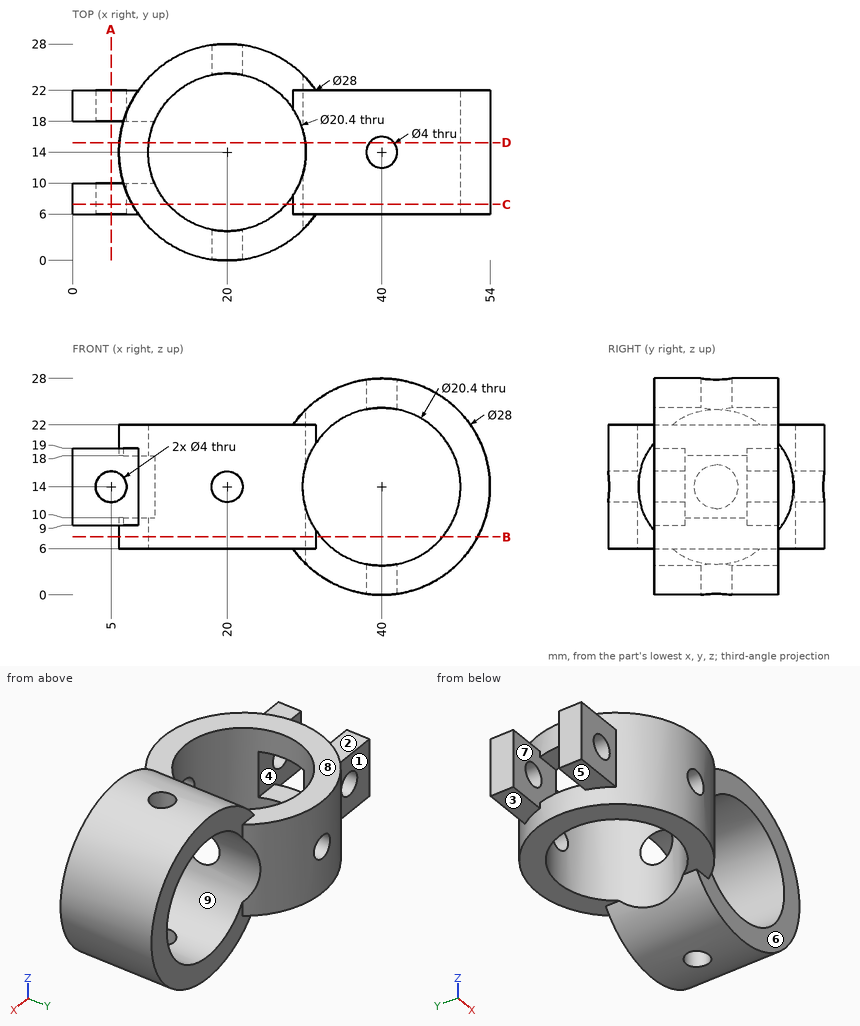
Geometry: see drawing. Coordinates: mm, zero at the bounding-box minimum. A direction names the side the tool comes from. Coordinates: 2 decimals unless noted, no trailing zeros. Loops run counter-clockwise (first coordinate to the right, second up) from the corner with the lowest first, then second, coordinate; pieces in that order, holes last. Notation, with made-up numbers: M 8,20.5 L 47,20.5 A16 cw 47,41.5 Z; hole C 2,22.25 d11. An arc over 180 degrees is marked long. Answer in a Markdown table with one row per item.
Q1. Draft query along Z for the marked faces 6, 7, 8 and 9. Return one class per face: pulls with the +Z half, pulls with the -Z half, needs draft (parallel to the pull), parting line crosses it, or undercut.
Answers below:
| item | result |
|---|---|
| face 6 | needs draft |
| face 7 | undercut |
| face 8 | pulls with the +Z half |
| face 9 | undercut |
Q2. Section B-B on z = 7.5. Return the cut outline in (x, y), plus the area to 3 significant figures.
Answers below:
| item | result |
|---|---|
| outline | M 31.49,6 L 32.14,6 L 32.14,22 L 31.49,22 A14 ccw long Z; M 47.86,6 L 52.4,6 L 52.4,22 L 47.86,22 Z; hole C 20,14 d20.4 |
| area | 345 mm^2 |
Q3. Section D-D on y = 15.25. Return the cut outline in (x, z).
Answers below:
| item | result |
|---|---|
| outline | M 6.06,6 L 9.88,6 L 9.88,10 L 6.06,10 Z; M 6.06,18 L 9.88,18 L 9.88,22 L 6.06,22 Z; M 30.12,4.08 A14 ccw 38.44,0.09 L 38.44,3.92 A10.2 cw 30.12,11.45 Z; M 30.12,16.55 A10.2 cw 38.44,24.08 L 38.44,27.91 A14 ccw 30.12,23.92 Z; M 41.56,0.09 A14 ccw 41.56,27.91 L 41.56,24.08 A10.2 cw 41.56,3.92 Z |
Q4. First-contact query: pin 1 (3.5 mm diameter, centred on x = 40, y = 14, fed in from -Z); pin 2 (7 mm diameter, centred on x = 6, z = 15.5, fed in from +Y); pin 3 (8 mm diameter, centred on x = 7, z = 13.5, fed in from +Y); pin 4 (8 mm diameter, centred on x = 14, z = 21.5, fed in from +Y). Flat tips, straight axial feed; report the tip coordinate or a pass-through.
Answers below:
| item | result |
|---|---|
| pin 1 | passes through |
| pin 2 | stops at y = 23.26 |
| pin 3 | stops at y = 24.72 |
| pin 4 | stops at y = 27.86 |
Q5. Section C-C on y = 7.25. Return the cut outline in (x, z), plus the area to 3 significant figures.
Answers below:
| item | result |
|---|---|
| outline | M 0,9 L 7.73,9 L 7.73,6 L 12.35,6 L 12.35,22 L 7.73,22 L 7.73,19 L 0,19 Z; M 27.65,6 L 28.51,6 A14 ccw long 28.51,22 L 27.65,22 Z; hole C 5,14 d4; hole C 40,14 d20.4 |
| area | 414 mm^2 |
Q6. Ray query, probe 1 along Z at (x, y) = (40, 11); probe 2 along Z at (x, y) = (5, 8.8); probe 3 along X at (y, z) = (25.25, 12.25). Return the intervals inside material, ascending. Write a range as from..to.
Answers below:
| item | result |
|---|---|
| probe 1 | z = 0..3.8, 24.2..28 |
| probe 2 | z = 9..12, 16..19 |
| probe 3 | x = 11.67..19.03, 20.97..28.33 |
Q7. Section A-A on x = 5. Return the cut outline in (y, z), plus the area to 3 significant figures.
Answers below:
| item | result |
|---|---|
| outline | M 6,9 L 10,9 L 10,12 L 6,12 Z; M 6,16 L 10,16 L 10,19 L 6,19 Z; M 18,9 L 22,9 L 22,12 L 18,12 Z; M 18,16 L 22,16 L 22,19 L 18,19 Z |
| area | 48.0 mm^2 |
Q8. Set-up query: the marked faces 1, 2, 3, 4 and 5. Return all of +Z, -Z, +X, -X, +Y, -Y with unobstructed straight access to the full face (end or side cutting, diameter ignored); none if empty.
Answers below:
| item | result |
|---|---|
| face 1 | +Z, -Z, -X, +Y |
| face 2 | +Z, -X, +Y |
| face 3 | -Z, -X, +Y |
| face 4 | -X |
| face 5 | -Z, -X, -Y |
